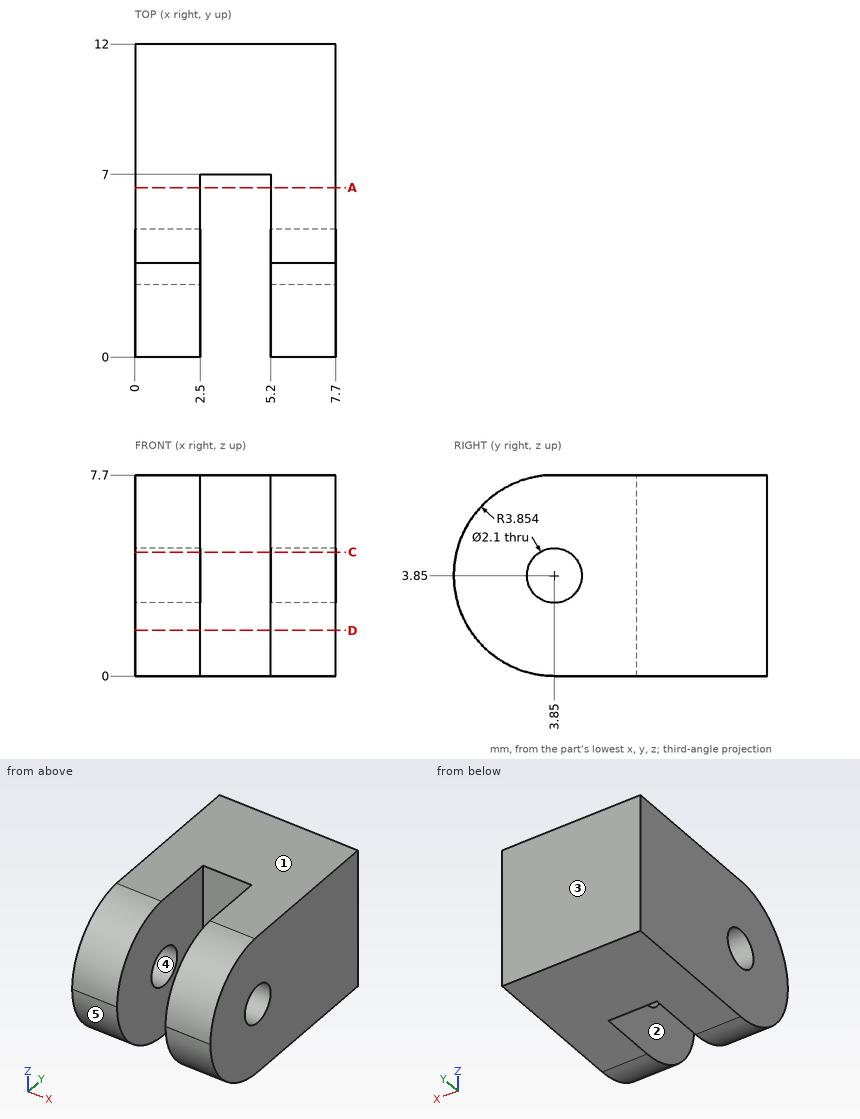
Source: three-view drawing plus pictorial views. Frame: mm from the lowest corner of the part. A direction names the side the tool comes from. Give positions to 0.01 mm unless a question says otherwise; leave off trailing zeros. Write each loop counter-clockwise with the first axis right and the second up, starting at its lowest first coordinate (ties: lowest second). Pieces come first, ordered by that corner, then holes. Notation, with made-up numbers: (-20.5, -15.5) - (26.5, -15.5) arc R38 cw to (26.5, 23.5) - close; hole circle Ø2 at (3, 71). An arc over 180 degrees is marked (long way). Write item = value, one per line. Start each with the question number.
1. Ray query, L1, parallel to Z at x = 5.7, y = 3.85; L2, parallel to X at y = 2, z = 3; L3, parallel to Y at x = 5.75, z = 4. Return the intervals inside material, ascending.
2. Section query A-A, the plane y = 6.5. Output: boundary loops of the cut face in (x, z), then the cut area to 3 significant figures.
3. Section query D-D, the plane z = 1.75. Output: boundary loops of the cut face in (x, y) (3 decimals).
4. Section query C-C, the plane z = 4.75. Output: boundary loops of the cut face in (x, y).
5. Access query for the marked faces 1 and 2. Directions: +Z, -Z, +X, -X, +Y, -Y. A direction counts if a zero-diameter tool reaches every point of the face in a straight line with its end or side. Return the directions, or none.
6. Mould query, pull axis Y, two halves, no side actions, for the marked faces 3, 4 and 5. Classes: released by +Y, released by -Y, zero draft, split by the parting line, or undercut.
7. First-contact query: pin 1 Ø3 at (x, z) = (3, 5.5) entering from -Y. Flat tip, straight axial feed; report the tip coordinate or a pass-through.
Check sheet entries:
q1.L1 = 0 to 2.8, 4.9 to 7.7
q1.L2 = 0 to 2.5, 5.2 to 7.7
q1.L3 = 0 to 2.81, 4.89 to 12
q2.outline = (0, 0) - (2.5, 0) - (2.5, 7.7) - (0, 7.7) - close; (5.2, 0) - (7.7, 0) - (7.7, 7.7) - (5.2, 7.7) - close
q2.area = 38.5 mm2
q3.outline = (0, 0.625) - (2.5, 0.625) - (2.5, 7) - (5.2, 7) - (5.2, 0.625) - (7.7, 0.625) - (7.7, 12) - (0, 12) - close
q4.outline = (0, 0.11) - (2.5, 0.11) - (2.5, 3.31) - (0, 3.31) - close; (0, 4.39) - (2.5, 4.39) - (2.5, 7) - (5.2, 7) - (5.2, 4.39) - (7.7, 4.39) - (7.7, 12) - (0, 12) - close; (5.2, 0.11) - (7.7, 0.11) - (7.7, 3.31) - (5.2, 3.31) - close
q5.face_1 = +Z, +X, -X, +Y, -Y
q5.face_2 = +Z, -Z, -Y
q6.face_3 = released by +Y
q6.face_4 = undercut
q6.face_5 = released by -Y
q7.pin_1 = 0.01
